The listing builds one solid part. Answer for the finished solid, in the listing's coordinates (mm). A direction names the side the tool comes from. Coordinates: 2 decimals unless noted, no trailing zeros. Write each loop counter-clockwise with the first axis right and the second up, starting at its lowest first coordinate (ties: lowest second). Pieces come first, ordered by that corner, then holes.
from build123d import *

# Parameters (mm, degrees)
F0_R            = 38.1
F1_DEPTH        = 12.7
F2_R            = 6.35
F3_DEPTH        = 12.701
F5_DEPTH        = 12.701
F5_COPIES_COUNT = 6


# Not quite as in the source:
# - a pattern or mirror of a feature is missing from the dataset's text; its kind, count and spacing are read off the source's solid


with BuildPart() as f1:
    # F0 (on Front) → F1 (new body)
    with BuildSketch(Plane.XZ):
        Circle(F0_R)
    extrude(amount=F1_DEPTH)

    # F2 (on face) → F3 (cut, through all)
    with BuildSketch(Plane.XZ.offset(12.7)):
        Circle(F2_R)
    extrude(amount=-F3_DEPTH, mode=Mode.SUBTRACT)

    # F4 (on face) → F5 (cut, through all)
    with BuildSketch(Plane.XZ.offset(12.7)):
        Polygon((0.8353452235, 14.3352959198), (7.9783069864, 20.7387890774), (4.0955196667, 29.5109376166), (-5.4471366308, 28.5289304107), (-7.4620352459, 19.149868041), align=None)
    f5 = extrude(amount=-F5_DEPTH, mode=Mode.SUBTRACT)

    # F5_copies: F5 ×6 about axis
    f5_copies_axis = Axis((0, 0, 0), (0, 1, 0))
    for i in range(1, F5_COPIES_COUNT):
        add(f5.rotate(f5_copies_axis, i * 360 / F5_COPIES_COUNT), mode=Mode.SUBTRACT)


solid = f1.part
1. Flat-ended cylindrical pins translate along their axes: P1, Ø1, axis at x = 10.5, y = -11, coming from the -Z side; P2, Ø5, axis at x = -14, y = -11, coming from the -Z side; P3, Ø4, axis at y = -3, z = -20, coming from the -X side. Find the tip coordinate at first contact, or state that the pin passes through.
Results found:
P1: stops at z = -36.76
P2: stops at z = -36.32
P3: stops at x = -33.58
2. A tool of negligible diameter and unlimited length cuts with its end or side. For faces 1 (the flat face through (8, 0, 1)), 2 (the flat face through (6.44, -6.44, -23.91)), from which of +Z, -Z, +X, -X, +Y, -Y can it reach the whole face along a straight path? Write none if from no direction.
Results found:
face 1: +Z, -Z, +X, -X, +Y
face 2: +Y, -Y
3. For a pull along Z with two mould halves and no side action, classify faces 3 (the flat face through (8, -12.7, 1)), 4 (the flat face through (-17.48, -6.44, -17.53)), 5 (the cylindrical face through (-30.235, -6.261, -23.183)) as pulls with the +Z half, pulls with the -Z half, needs draft (parallel to the pull), parting line crosses it, or undercut.
Results found:
face 3: needs draft
face 4: undercut
face 5: parting line crosses it
4. Section A-A on z = 0 is taken. Give the vertices of the cut face in (x, y).
Results found:
outline: (-38.1, -12.7) - (-6.35, -12.7) - (-6.35, 0) - (-38.1, 0) - close; (6.35, -12.7) - (38.1, -12.7) - (38.1, 0) - (6.35, 0) - close
5. Section B-B on y = -2.25 is taken. State how many separate pieces and enclosed holes the cut face has, then the cut area to 3 significant figures.
Results found:
separate pieces: 1
enclosed holes: 7
area: 3,480 mm2
6. Section C-C on x = -25 is taken. Give the vertices of the cut face in (y, z).
Results found:
outline: (-12.7, -28.75) - (0, -28.75) - (0, -14.81) - (-12.7, -14.81) - close; (-12.7, -7.64) - (0, -7.64) - (0, 7.35) - (-12.7, 7.35) - close; (-12.7, 14.97) - (0, 14.97) - (0, 28.75) - (-12.7, 28.75) - close
7. Find the intervals of material crossed by L1, parallel to X at y = -8.5, z = -6.5; L2, parallel to Z at x = 0, y = -5.5; L3, parallel to Z at x = 24.5, y = -10, in increasing order.
Results found:
L1: x = -37.54 to -24.17, -12.83 to 14.42, 24.06 to 37.54
L2: z = -38.1 to -29.09, -14.82 to -6.35, 6.35 to 14.82, 29.09 to 38.1
L3: z = -29.18 to -16.09, -6.9 to 6.95, 15.5 to 29.18
